Source: CAD feature listing. Evaluate the final solid. Frame: model axes, mm. A direction names the side the tool comes from. Give positions to 0.01 mm unless a question says otherwise; leave off trailing zeros. Write each loop counter-clockwise with the first axis right and the second up, starting at its lowest first coordinate (ties: lowest second). Pieces come first, ordered by that corner, then holes. Notation, with made-up numbers: M 8,34.25 L 27,34.25 A17 ccw 27,46.25 Z; hole C 57.5,-36.75 d8. An arc over 180 degrees is marked long. Use CSV: the item, a comma, the result in double quotes. Start each with the question number.
from build123d import *

# Parameters (mm, degrees)
F0_W     = 56.8
F0_H     = 56.8
F1_DEPTH = 32
F2_T     = -2.5
F3_R     = 1.5
F4_DEPTH = 2.5
F5_SIZE  = 2.49999


# Not quite as in the source:
# - a fillet or chamfer is up to 0.001 mm smaller than in the source, because OpenCascade refuses the exact size


with BuildPart() as f1:
    # F0 (on Top) → F1 (new body)
    with BuildSketch(Plane.XY):
        with Locations((28.4, 28.4)):
            Rectangle(F0_W, F0_H)
    extrude(amount=F1_DEPTH)

    # F2
    f2_openings = [f1.faces().sort_by_distance(p)[0] for p in [
        (28.4, 28.4, 32),
    ]]
    offset(amount=F2_T, openings=f2_openings)

    # F3 (on face) → F4 (cut, through all)
    with BuildSketch(Plane(origin=(0, 0, 0), x_dir=(1, 0, 0), z_dir=(0, 0, -1))):
        with Locations((25.4, -28.4)):
            Circle(F3_R)
        with Locations((31.4, -28.4)):
            Circle(F3_R)
    extrude(amount=-F4_DEPTH, mode=Mode.SUBTRACT)

    # F5 (size 2.5 in the source; OpenCascade refuses exactly that, so slightly less here)
    f5_edges = [f1.edges().sort_by_distance(p)[0] for p in [
        (2.5, 28.4, 32),
        (28.4, 2.5, 32),
        (54.3, 28.4, 32),
        (28.4, 54.3, 32),
    ]]
    chamfer(f5_edges, length=F5_SIZE)


solid = f1.part
1. Section C-C on z = 23. Return loops of the section in (x, y).
2. First-contact query: pin 1 (4 mm diameter, centred on x = 25.4, y = 28.4, fed in from +Z). Flat tip, straight axial feed; report the tip coordinate or a pass-through.
3. Section B-B on y = 28.4. Give the number of separate pieces and of enclosed holes in the cut face, then the cut area to 3 significant figures.
4. Line query: probe 1 along X at (y, z) = (28.4, 1.1); probe 2 along X at (y, z) = (6.5, 13). Output: solid intervals per line, ascending.
5. Access query for faces 5 (the cylindrical face through (26.09, 29.73, 1.23)), 6 (the flat face through (1, 28, 31)). Directions: +Z, -Z, +X, -X, +Y, -Y. A direction counts if a zero-diameter tool reaches every point of the face in a straight line with its end or side. Return the directions, or none.
6. Pull-direction query (X, two-part tool) for faces 1 (the flat face through (28, 55.5, 30.7)), 2 (the flat face through (28, 0, 16)), 3 (the cylindrical face through (32.09, 29.73, 1.23)), 4 (the flat face through (0, 28, 16)); classes: released by +X, released by -X, zero draft, split by the parting line, or undercut.
Resolved:
1,outline,"M 0,0 L 56.8,0 L 56.8,56.8 L 0,56.8 Z; hole M 2.5,2.5 L 54.3,2.5 L 54.3,54.3 L 2.5,54.3 Z"
2,pin 1,"stops at z = 2.5"
3,separate pieces,"3"
3,enclosed holes,"0"
3,area,"268 mm2"
4,probe 1,"x = 0 to 23.9, 26.9 to 29.9, 32.9 to 56.8"
4,probe 2,"x = 0 to 2.5, 54.3 to 56.8"
5,face 5,"+Z, -Z"
5,face 6,"+Z"
6,face 1,"undercut"
6,face 2,"zero draft"
6,face 3,"undercut"
6,face 4,"released by -X"
